```python
from build123d import *

# Parameters (mm, degrees)
SKETCH1_W           = 150
SKETCH1_H           = 150
BOSS_EXTRUDE1_DEPTH = 40
SKETCH2_W           = 130
SKETCH2_H           = 130
CUT_EXTRUDE1_DEPTH  = 54
SKETCH6_R           = 2.5
BOSS_EXTRUDE5_DEPTH = 5
SKETCH9_R           = 1.4
CUT_EXTRUDE4_DEPTH  = 10
CIRPATTERN1_COUNT   = 3
CIRPATTERN1_ANGLE   = 180
SKETCH10_W          = 130
SKETCH10_H          = 96.398295943
CUT_EXTRUDE6_DEPTH  = 46


with BuildPart() as part:
    # Sketch1 → Boss-Extrude1 (new body)
    with BuildSketch(Plane(origin=(0, 0, 0), x_dir=(1, 0, 0), z_dir=(0, 1, 0))):
        Rectangle(SKETCH1_W, SKETCH1_H)
    extrude(amount=-BOSS_EXTRUDE1_DEPTH)

    # Sketch2 → Cut-Extrude1 (cut)
    with BuildSketch(Plane(origin=(0, 0, 0), x_dir=(1, 0, 0), z_dir=(0, 1, 0))):
        Rectangle(SKETCH2_W, SKETCH2_H)
    extrude(amount=-CUT_EXTRUDE1_DEPTH, mode=Mode.SUBTRACT)

    # Sketch6 → Boss-Extrude5 (add)
    with BuildSketch(Plane.XZ.offset(40)):
        with Locations((-70.678187872, -25)):
            Circle(SKETCH6_R)
        with Locations((-70.678187872, 25)):
            Circle(SKETCH6_R)
        with Locations((25, 70.678187872)):
            Circle(SKETCH6_R)
        with Locations((-25, 70.678187872)):
            Circle(SKETCH6_R)
        with Locations((70.678187872, -25)):
            Circle(SKETCH6_R)
        with Locations((70.678187872, 25)):
            Circle(SKETCH6_R)
        with Locations((-25, -70.678187872)):
            Circle(SKETCH6_R)
        with Locations((25, -70.678187872)):
            Circle(SKETCH6_R)
    extrude(amount=BOSS_EXTRUDE5_DEPTH)

    # Sketch9 → Cut-Extrude4 (cut)
    with BuildSketch(Plane.ZY.offset(75)):
        with Locations((-6.1, -7.25)):
            Circle(SKETCH9_R)
        with Locations((6.1, -7.25)):
            Circle(SKETCH9_R)
        with Locations((6.1, -15.25)):
            Circle(SKETCH9_R)
        with Locations((-6.1, -15.25)):
            Circle(SKETCH9_R)
    cut_extrude4 = extrude(amount=-CUT_EXTRUDE4_DEPTH, mode=Mode.SUBTRACT)

    # CirPattern1: Cut-Extrude4 ×3 about axis
    cirpattern1_axis = Axis((0, 0, 0), (0, 1, 0))
    for i in range(1, CIRPATTERN1_COUNT):
        add(cut_extrude4.rotate(cirpattern1_axis, i * CIRPATTERN1_ANGLE / (CIRPATTERN1_COUNT - 1)), mode=Mode.SUBTRACT)

    # Sketch10 → Cut-Extrude6 (cut, through all)
    with BuildSketch(Plane(origin=(0, 0, 0), x_dir=(1, 0, 0), z_dir=(0, 1, 0))):
        with Locations((0, 113.199147972)):
            Rectangle(SKETCH10_W, SKETCH10_H)
    extrude(amount=-CUT_EXTRUDE6_DEPTH, mode=Mode.SUBTRACT)


solid = part.part
```
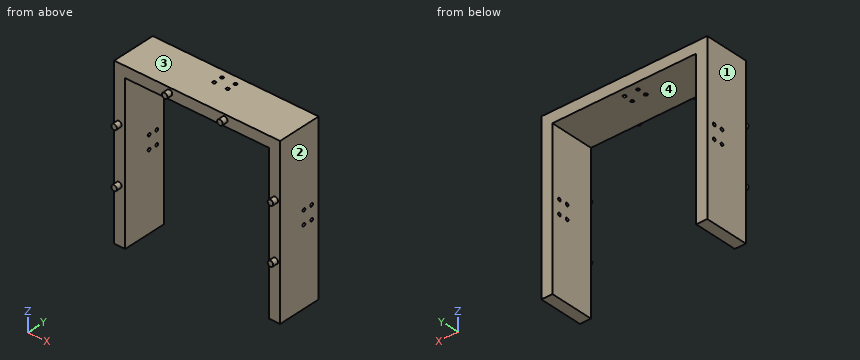
Could you check a few things on this model? Use its own coordinates, in mm. Face numbers are marked on the shaded views. Round coordinates to 2 decimals unless told otherwise and drop trailing zeros. Loops run counter-clockwise (first coordinate to the right, second up) from the corner with the lowest first, then second, coordinate; pieces in that order, holes last. Notation, with made-up numbers: (33.25, 78.5) -> (59.25, 78.5) arc R16 cw to (59.25, 93.5) -> close; hole circle Ø3 at (18.25, 79.25). An arc over 180 degrees is marked (long way). Put each result on its own line as item: value.
Q1. I want a section at D-D on z = -25. Write out the boundary of the cut face in (x, y), and give its area (3 significant figures).
Checks:
outline: (-75, -40) -> (-73.18, -40) -> (-73.18, -45) -> (-68.18, -45) -> (-68.18, -40) -> (-65, -40) -> (-65, 0) -> (-75, 0) -> close; (65, -40) -> (68.18, -40) -> (68.18, -45) -> (73.18, -45) -> (73.18, -40) -> (75, -40) -> (75, 0) -> (65, 0) -> close
area: 850 mm2
Q2. I want a section at B-B on x = 25. Write out the boundary of the cut face in (y, z), and give its area (3 significant figures).
Checks:
outline: (-45, 68.18) -> (-40, 68.18) -> (-40, 65) -> (0, 65) -> (0, 75) -> (-40, 75) -> (-40, 73.18) -> (-45, 73.18) -> close
area: 425 mm2
Q3. For pin 1 Ø20 at (x, y) = (-30.5, -27) entering from -Z; pin 2 Ø2 at (x, y) = (6.1, -7.25) entering from +Z, each with a flat end and sliding along its axis, tell me the tip position at first contact or that it passes through.
Checks:
pin 1: z = 65
pin 2: through
Q4. I want a section at A-A on z = 31. Write out the boundary of the cut face in (x, y).
Checks:
outline: (-75, -40) -> (-65, -40) -> (-65, 0) -> (-75, 0) -> close; (65, -40) -> (75, -40) -> (75, 0) -> (65, 0) -> close
Q5. Please list where these lines run through material, in increasing order: line 1 (Y direction, x = 6.1, z = 72); line 2 (Z direction, x = -69, y = -7). Write a range as from..to.
Checks:
line 1: -40..-16.65, -13.85..-8.65, -5.85..0
line 2: -75..-7.48, -4.72..4.72, 7.48..75
Q6. I want a section at C-C on y = -34. Write out the boundary of the cut face in (x, z), and give its area (3 significant figures).
Checks:
outline: (-75, -75) -> (-65, -75) -> (-65, 65) -> (65, 65) -> (65, -75) -> (75, -75) -> (75, 75) -> (-75, 75) -> close
area: 4,300 mm2
Q7. Thinking about a two-plate mould opening in X: for the marked faces 1, 2, 3 and 4, which applies, pulls with the +X half, pulls with the -X half, needs draft (parallel to the pull), parting line crosses it, or undercut?
Checks:
face 1: pulls with the -X half
face 2: pulls with the +X half
face 3: needs draft
face 4: undercut
